CAD build for the part. Positions are in the model's coordinates, mm. A direction names the side the tool comes from. Give positions to 0.01 mm unless a question says otherwise; leave off trailing zeros. Order: outer loops, then holes, each group sorted by start corner. A loop starts at its lowest first (then second) coordinate and runs counter-clockwise, first axis right, second up. Notation, with made-up numbers: M -37.5,-31.75 L 19.5,-31.75 A4 cw 19.5,-25.75 Z; hole C 2,34 d10. An arc over 180 degrees is marked long. Put each result on its own line as item: value. Start each with the question number.
1) Pin check, flat tips, straight feed: pin 1 (8 mm diameter, centred on x = 25, y = 25, fed in from +Z); pin 2 (1 mm diameter, centred on x = 51, z = 2.5, fed in from -Y); pin 3 (1.5 mm diameter, centred on x = 49.5, z = 1.5, fed in from -Y). Stop position of each tip, or through.
2) Cut at B-B (y = 34). Write the cut outline in (x, z).
3) Cut at A-A (z = 1.35). Give the number of separate pieces and of enclosed holes in the cut face, and give its area (3 significant figures).
4) Two-plate mould, pull along X, no slides. Class faces 1 (the face through (46.99, 47.15, 1.48)), 2 (the face through (3.01, 2.85, 1.48)), 3 (the face through (41.526, 8.352, 1.479)): released by +X, released by -X, zero draft, split by the parting line, or undercut.
5) Tool access for faces 4 (the face through (63, 10, 1)), 5 (the face through (43, 41, 1)), 6 (the face through (62, 40, 1)): list every direction of +Z, -Z, +X, -X, +Y, -Y with a clear straight run to the whole face (end or side of a thin tool).
6) Cut at D-D (x = 64.5). Write the cut outline in (y, z), and give its area (3 significant figures).
7) Cut at C-C (x = 7). Write the cut outline in (y, z), and give its area (3 significant figures).
8) Drill centre lines: line 1 (Y direction, x = 25, z = 1.45); line 2 (Y direction, x = 6, z = 1.25); line 3 (Y direction, x = 7, z = 1.9). Where is each one in solid material? Low to high. Write a range as [from, to].
```python
from build123d import *

# Parameters (mm, degrees)
CROQUIS1_R              = 2.5
CROQUIS1_R_2            = 2
SALIENTE_EXTRUIR1_DEPTH = 3


with BuildPart() as part:
    # Croquis1 → Saliente-Extruir1 (new body)
    with BuildSketch(Plane.XY):
        with BuildLine():
            ThreePointArc((0, 40), (2.928932188, 47.071067812), (10, 50))
            Line((10, 50), (40, 50))
            ThreePointArc((40, 50), (47.071067812, 47.071067812), (50, 40))
            Line((50, 40), (50, 10))
            ThreePointArc((50, 10), (47.071067812, 2.928932188), (40, 0))
            Line((40, 0), (10, 0))
            ThreePointArc((10, 0), (2.928932188, 2.928932188), (0, 10))
            Line((0, 10), (0, 40))
        make_face()
        with Locations((45, 35)):
            Circle(CROQUIS1_R, mode=Mode.SUBTRACT)
        with Locations((25, 25)):
            Circle(CROQUIS1_R, mode=Mode.SUBTRACT)
        with Locations((43, 43)):
            Circle(CROQUIS1_R_2, mode=Mode.SUBTRACT)
        with Locations((7, 43)):
            Circle(CROQUIS1_R_2, mode=Mode.SUBTRACT)
        with Locations((43, 7)):
            Circle(CROQUIS1_R_2, mode=Mode.SUBTRACT)
        with Locations((7, 7)):
            Circle(CROQUIS1_R_2, mode=Mode.SUBTRACT)
        with BuildLine():
            ThreePointArc((75, 40), (78.535533906, 38.535533906), (80, 35))
            Line((80, 35), (80, 15))
            ThreePointArc((80, 15), (78.535533906, 11.464466094), (75, 10))
            Line((75, 10), (50, 10))
            Line((50, 10), (50, 40))
            Line((50, 40), (75, 40))
        make_face()
        with Locations((70, 16)):
            Circle(CROQUIS1_R_2, mode=Mode.SUBTRACT)
        with Locations((70, 34)):
            Circle(CROQUIS1_R_2, mode=Mode.SUBTRACT)
    extrude(amount=SALIENTE_EXTRUIR1_DEPTH)


solid = part.part
```
Solution:
1. pin 1: z = 3
1. pin 2: y = 10
1. pin 3: y = 5.16
2. outline: M 0,0 L 42.71,0 L 42.71,3 L 0,3 Z; M 47.29,0 L 68,0 L 68,3 L 47.29,3 Z; M 72,0 L 80,0 L 80,3 L 72,3 Z
3. separate pieces: 1
3. enclosed holes: 8
3. area: 3,190 mm²
4. face 1: released by +X
4. face 2: released by -X
4. face 3: undercut
5. face 4: +Z, -Z, +X, -Y
5. face 5: +Z, -Z
5. face 6: +Z, -Z, +X, +Y
6. outline: M 10,0 L 40,0 L 40,3 L 10,3 Z
6. area: 90.0 mm²
7. outline: M 0.46,0 L 5,0 L 5,3 L 0.46,3 Z; M 9,0 L 41,0 L 41,3 L 9,3 Z; M 45,0 L 49.54,0 L 49.54,3 L 45,3 Z
7. area: 123 mm²
8. line 1: [0, 22.5], [27.5, 50]
8. line 2: [0.83, 5.27], [8.73, 41.27], [44.73, 49.17]
8. line 3: [0.46, 5], [9, 41], [45, 49.54]
